Geometry check sheet. Reference: the model listing, model coordinates, mm. A direction names the side the tool comes from. Coordinates: 2 decimals unless noted, no trailing zeros. Order: outer loops, then holes, each group sorted by start corner. A loop starts at its lowest first (then second) coordinate and runs counter-clockwise, first axis right, second up. Notation, with made-up numbers: (74.5, -12.75) - (128.5, -12.75) arc R27 ccw to (128.5, 7.25) - close; hole circle Ø5 at (8.25, -32.75). An arc over 180 degrees is marked (long way). Put each result on its own line as item: value.
from build123d import *

# Parameters (mm, degrees)
SKETCH1_W            = 45
SKETCH1_H            = 39
BOSS_EXTRUDE1_DEPTH  = 22
M4_CLEARANCE_HOLE1_D = 4.3
SKETCH5_R            = 3.8
CUT_EXTRUDE1_DEPTH   = 16.2


with BuildPart() as part:
    # Sketch1 → Boss-Extrude1 (new body)
    with BuildSketch(Plane(origin=(0, 0, 0), x_dir=(1, 0, 0), z_dir=(0, 1, 0))):
        Rectangle(SKETCH1_W, SKETCH1_H)
    extrude(amount=BOSS_EXTRUDE1_DEPTH)

    # M4 Clearance Hole1 (through all)
    with Locations(Plane(origin=(0, 0, 0), x_dir=(-1, 0, 0), z_dir=(0, -1, 0))):
        with Locations((0, -14.65), (-17.95, 14.65), (17.95, 14.65)):
            Hole(M4_CLEARANCE_HOLE1_D / 2)

    # Sketch5 → Cut-Extrude1 (cut)
    with BuildSketch(Plane(origin=(0, 22, 0), x_dir=(1, 0, 0), z_dir=(0, 1, 0))):
        with Locations(Location((0, -14.65, 0), (0, 0, 270))):
            Circle(SKETCH5_R)
        with BuildLine():
            Line((-14.15, 14.65), (-14.15, 22.25))
            Line((-14.15, 22.25), (-25.55, 22.25))
            Line((-25.55, 22.25), (-25.55, 10.85))
            Line((-25.55, 10.85), (-17.95, 10.85))
            ThreePointArc((-17.95, 10.85), (-15.262994231, 11.962994231), (-14.15, 14.65))
        make_face()
        with BuildLine():
            Line((17.95, 10.85), (25.55, 10.85))
            Line((25.55, 10.85), (25.55, 22.25))
            Line((25.55, 22.25), (14.15, 22.25))
            Line((14.15, 22.25), (14.15, 14.65))
            ThreePointArc((14.15, 14.65), (15.262994231, 11.962994231), (17.95, 10.85))
        make_face()
    extrude(amount=-CUT_EXTRUDE1_DEPTH, mode=Mode.SUBTRACT)


solid = part.part
Q1. Thickness scan on L1, parallel to X at y = 1.5, z = -14.65; L2, parallel to Z at x = 18, y = 14.5; L3, parallel to X at y = 9.75, z = 12.5. Record the ranges inside material, lowest first. Write a range as [from, to].
Answer block:
L1: x = [-22.5, -20.1], [-15.8, 15.8], [20.1, 22.5]
L2: z = [-10.85, 19.5]
L3: x = [-22.5, -3.13], [3.13, 22.5]
Q2. Section check D-D on x = -18.5. Record the boundary of the cut face in (y, z), then the cut area to 3 significant figures.
Answer block:
outline: (0, -19.5) - (5.8, -19.5) - (5.8, -16.73) - (0, -16.73) - close; (0, -12.57) - (5.8, -12.57) - (5.8, -10.85) - (22, -10.85) - (22, 19.5) - (0, 19.5) - close
area: 694 mm^2
Q3. Section check C-C on y = 16.25. Record the boundary of the cut face in (x, z).
Answer block:
outline: (-22.5, -10.85) - (-17.95, -10.85) arc R3.8 cw to (-14.15, -14.65) - (-14.15, -19.5) - (14.15, -19.5) - (14.15, -14.65) arc R3.8 cw to (17.95, -10.85) - (22.5, -10.85) - (22.5, 19.5) - (-22.5, 19.5) - close; hole circle Ø7.6 at (0, 14.65)
Q4. Depth check by flat-ended pin: pin 1 Ø1.4 at (x, y) = (-19.5, 17) entering from -Z; pin 2 Ø5.5 at (x, z) = (0, 14.65) entering from -Y; pin 3 Ø1.5 at (y, z) = (16, -16) entering from -X; pin 4 Ø2.5 at (x, z) = (1.5, 16.5) entering from +Y. Enter the tip coordinate at first touch or a pass-through.
Answer block:
pin 1: stops at z = -10.85
pin 2: stops at y = 0
pin 3: stops at x = -14.15
pin 4: stops at y = 5.8
Q5. Section check B-B on x = 0. Record the boundary of the cut face in (y, z), then the cut area to 3 significant figures.
Answer block:
outline: (0, -19.5) - (22, -19.5) - (22, 10.85) - (5.8, 10.85) - (5.8, 12.5) - (0, 12.5) - close; (0, 16.8) - (5.8, 16.8) - (5.8, 18.45) - (22, 18.45) - (22, 19.5) - (0, 19.5) - close
area: 710 mm^2
Q6. Access from +Z, -Z, +X, -X, +Y, -Y to the whole of each face (thin tool, end or side, straight path). Record for faces 1 (the flat face through (18, 5.8, -17)), 2 (the cylindrical face through (19.11, 2.94, -16.46)), 3 (the flat face through (-20.2, 5.8, -15.2)), 4 (the cylindrical face through (1.141, 14.013, 18.275)).
Answer block:
face 1: -Z, +X, +Y
face 2: +Y, -Y
face 3: -Z, -X, +Y
face 4: +Y
Q7. Section check A-A on y = 4.5. Record the boundary of the cut face in (x, z).
Answer block:
outline: (-22.5, -19.5) - (22.5, -19.5) - (22.5, 19.5) - (-22.5, 19.5) - close; hole circle Ø4.3 at (-17.95, -14.65); hole circle Ø4.3 at (0, 14.65); hole circle Ø4.3 at (17.95, -14.65)
